Part print with two shaded views. Sizes in mm from the minimum x, y, z corner. A direction names the side the tool comes from. Round coordinates to 2 decimals unless told otherwise and drop trailing zeros. Loops run counter-clockwise (first coordinate to the right, second up) from the corner with the lowest first, then second, coordinate; pieces in that order, holes last. Notation, with made-up numbers: (16.5, 86.25) - (47.5, 86.25) arc R29 cw to (47.5, 106.25) - close; hole circle Ø5 at (21, -32). An arc over 180 degrees is marked (long way). Use a Markdown table: item, result.
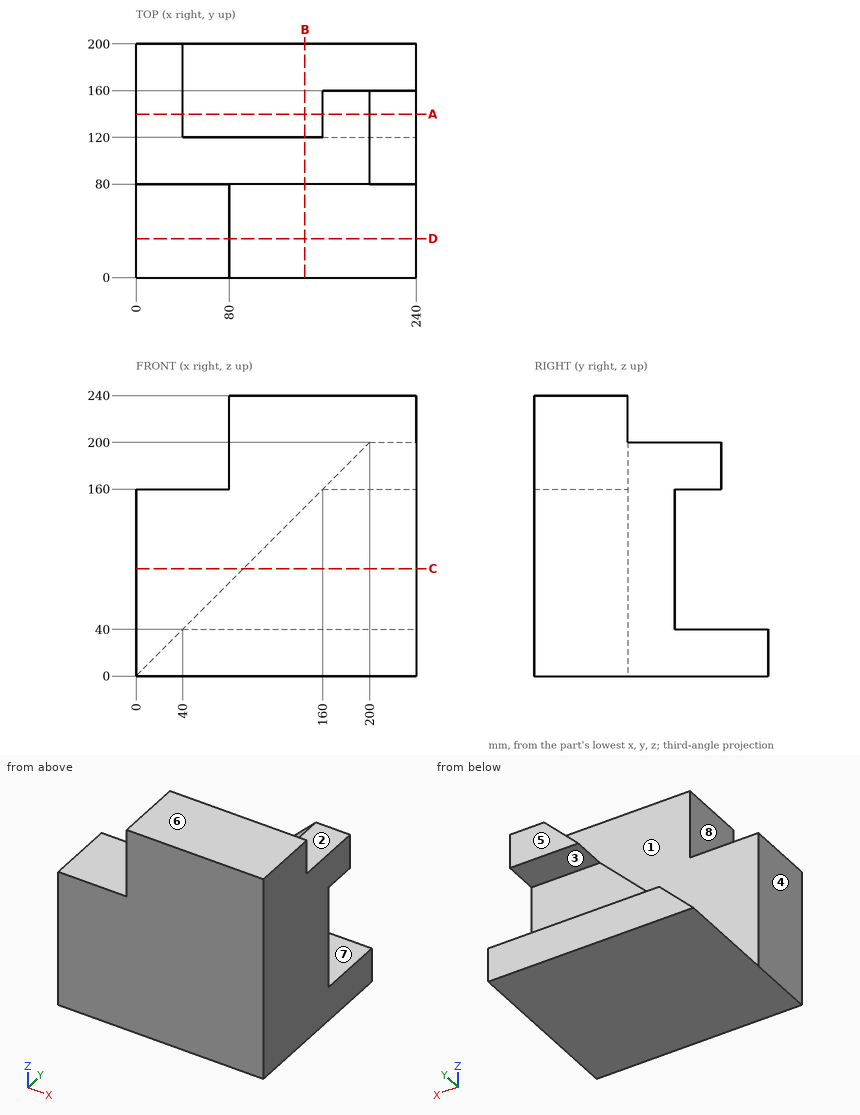
Q1. Cut at B-B, the plane x = 144.5. List the corners of the cut face in (y, z), plus the area to 3 significant figures.
Results found:
| item | result |
|---|---|
| outline | (0, 0) - (200, 0) - (200, 40) - (120, 40) - (120, 144.5) - (80, 144.5) - (80, 240) - (0, 240) - close |
| area | 28,200 mm2 |
Q2. Pull direction Z, two halves, no side cores. Call the marked faces 1, 2 and 3: pulls with the +Z half, pulls with the -Z half, needs draft (parallel to the pull), parting line crosses it, or undercut.
Results found:
| item | result |
|---|---|
| face 1 | needs draft |
| face 2 | pulls with the +Z half |
| face 3 | undercut |
Q3. Which spindle directions (+Z, -Z, +X, -X, +Y, -Y) get a long thin tool onto all of the face, cutting with end or side? Do the marked faces 4, 5, 6, 7 and 8. Say none if no direction does.
Results found:
| item | result |
|---|---|
| face 4 | +Z, -Z, -X, +Y, -Y |
| face 5 | +Z, +X, -X, +Y |
| face 6 | +Z, +X, -X, +Y, -Y |
| face 7 | +X, -X, +Y |
| face 8 | +Z, -X, +Y, -Y |
Q4. Drop flat-ended pins along their axis: pin 1 (12 mm diameter, centred on x = 189, y = 159.5, fed in from +Z); pin 2 (12 mm diameter, centred on x = 211.5, y = 120, fed in from +Z); pin 3 (4 mm diameter, centred on x = 63.5, z = 55.5, fed in from +Y); pin 4 (8 mm diameter, centred on x = 96.5, y = 113, fed in from -Z). Give the stop position or say it passes through.
Results found:
| item | result |
|---|---|
| pin 1 | stops at z = 195 |
| pin 2 | stops at z = 200 |
| pin 3 | stops at y = 120 |
| pin 4 | stops at z = 0 |
Q5. Cut at A-A, the plane y = 140. List the corners of the cut face in (x, z), plus the area to 3 significant figures.
Results found:
| item | result |
|---|---|
| outline | (0, 0) - (240, 0) - (240, 40) - (40, 40) - close; (160, 160) - (240, 160) - (240, 200) - (200, 200) - close |
| area | 11,200 mm2 |
Q6. Cut at D-D, the plane y = 33.5. List the corners of the cut face in (x, z), plus the area to 3 significant figures.
Results found:
| item | result |
|---|---|
| outline | (0, 0) - (240, 0) - (240, 240) - (80, 240) - (80, 160) - (0, 160) - close |
| area | 51,200 mm2 |
Q7. Probe line 1 (Y direction, x = 29, z = 31); line 2 (Z direction, x = 44, y = 151); line 3 (X direction, y = 105.5, z = 40). List the from-to ranges inside material, lowest first.
Results found:
| item | result |
|---|---|
| line 1 | y = 0 to 80 |
| line 2 | z = 0 to 40 |
| line 3 | x = 40 to 240 |
Q8. Cut at C-C, the plane z = 92. List the corners of the cut face in (x, y), plus the area to 3 significant figures.
Results found:
| item | result |
|---|---|
| outline | (0, 0) - (240, 0) - (240, 120) - (92, 120) - (92, 80) - (0, 80) - close |
| area | 25,100 mm2 |
